from build123d import *

# Parameters (mm, degrees)
SKETCH_1_R               = 37.5
SKETCH_1_R_2             = 35.5
EXTRUDE_1_DEPTH          = 214
SKETCH_2_R               = 1.5
CUT_EXTRUDE_1_DEPTH      = 88
PATTERN_CIRCULAR_1_COUNT = 3
SKETCH_3_W               = 5
SKETCH_3_H               = 20.375275098
CUT_EXTRUDE_2_DEPTH      = 2
PATTERN_CIRCULAR_2_COUNT = 3
SKETCH_4_W               = 5
SKETCH_4_H               = 20.375275098
CUT_EXTRUDE_3_DEPTH      = 2
PATTERN_CIRCULAR_3_COUNT = 3
CUT_EXTRUDE_4_DEPTH      = 156
CUT_EXTRUDE_4_DEPTH_BACK = 165
SKETCH_5_W               = 164.762813688
SKETCH_5_H               = 214


with BuildPart() as part:
    # Эскиз1 → Бобышка-Вытянуть1 (new body)
    with BuildSketch(Plane.XY):
        Circle(SKETCH_1_R)
        Circle(SKETCH_1_R_2, mode=Mode.SUBTRACT)
    extrude(amount=EXTRUDE_1_DEPTH)

    # Эскиз2 → Вырез-Вытянуть1 (cut)
    with BuildSketch(Plane(origin=(0, 0, 0), x_dir=(1, 0, 0), z_dir=(0, 1, 0))):
        with Locations(Location((0, -5, 0), (0, 0, 270))):
            Circle(SKETCH_2_R)
        with Locations(Location((0, -209, 0), (0, 0, 270))):
            Circle(SKETCH_2_R)
    cut_extrude_1 = extrude(amount=-CUT_EXTRUDE_1_DEPTH, mode=Mode.SUBTRACT)

    # Круговой массив1: Вырез-Вытянуть1 ×3 about axis
    pattern_circular_1_axis = Axis((0, 0, 214), (0, 0, -1))
    for i in range(1, PATTERN_CIRCULAR_1_COUNT):
        add(cut_extrude_1.rotate(pattern_circular_1_axis, i * 360 / PATTERN_CIRCULAR_1_COUNT), mode=Mode.SUBTRACT)

    # Эскиз3 → Вырез-Вытянуть2 (cut)
    with BuildSketch(Plane(origin=(0, 0, 0), x_dir=(-1, 0, 0), z_dir=(0, 0, -1))):
        with Locations((0, 27.321603857)):
            Rectangle(SKETCH_3_W, SKETCH_3_H)
    cut_extrude_2 = extrude(amount=-CUT_EXTRUDE_2_DEPTH, mode=Mode.SUBTRACT)

    # Круговой массив2: Вырез-Вытянуть2 ×3 about axis
    pattern_circular_2_axis = Axis((0, 0, 0), (0, 0, 1))
    for i in range(1, PATTERN_CIRCULAR_2_COUNT):
        add(cut_extrude_2.rotate(pattern_circular_2_axis, i * 360 / PATTERN_CIRCULAR_2_COUNT), mode=Mode.SUBTRACT)

    # Эскиз4 → Вырез-Вытянуть3 (cut)
    with BuildSketch(Plane.XY.offset(214)):
        with Locations((0, 27.321603857)):
            Rectangle(SKETCH_4_W, SKETCH_4_H)
    cut_extrude_3 = extrude(amount=-CUT_EXTRUDE_3_DEPTH, mode=Mode.SUBTRACT)

    # Круговой массив3: Вырез-Вытянуть3 ×3 about axis
    pattern_circular_3_axis = Axis((0, 0, 0), (0, 0, 1))
    for i in range(1, PATTERN_CIRCULAR_3_COUNT):
        add(cut_extrude_3.rotate(pattern_circular_3_axis, i * 360 / PATTERN_CIRCULAR_3_COUNT), mode=Mode.SUBTRACT)

    # Эскиз5 → Вырез-Вытянуть4 (cut, two sides: drawn at the far end of the back side and taken through both)
    with BuildSketch(Plane(origin=(0, 0, 0), x_dir=(1, 0, 0), z_dir=(0, 1, 0)).offset(-CUT_EXTRUDE_4_DEPTH_BACK)):
        Rectangle(SKETCH_5_W, SKETCH_5_H)
    extrude(amount=CUT_EXTRUDE_4_DEPTH + CUT_EXTRUDE_4_DEPTH_BACK, mode=Mode.SUBTRACT)


solid = part.part
Could you check a few things on this model? Use its own coordinates, in mm. A direction names the side the tool comes from. Give positions to 0.01 mm unless a question says otherwise; leave off trailing zeros. Loops run counter-clockwise (first coordinate to the right, second up) from the corner with the lowest first, then second, coordinate; pieces in that order, holes last. Notation, with made-up numbers: (77, 30.25) -> (127, 30.25) arc R22 cw to (127, 67.25) -> close; hole circle Ø4 at (-30.75, -22). An arc over 180 degrees is marked (long way). Return JSON: item names as keys, results as strings.
Item 1: Which directions (+Z, -Z, +X, -X, +Y, -Y) give clear straight access to the entire face, cutting with the end or side of a thin tool? Please do faces 1 (the flat face through (-30.5, 18.6, 214)), 2 (the flat face through (32, -18, 212)), 3 (the cylindrical face through (-0.575, -36.47, 210.386)).
Geometry results:
{"face 1": "+Z, +X, -X, +Y, -Y", "face 2": "+Z", "face 3": "-Y"}
Item 2: I'm going to push flat-ended pins straight in: pin 1 (3.5 mm diameter, centred on x = 31.5, y = -17.5, fed in from +Z); pin 2 (1 mm diameter, centred on y = 8, z = 153.5, fed in from +X); pin 3 (8 mm diameter, centred on y = -27, z = 175.5, fed in from -X). Where does each tip first touch, or does it pass through?
Geometry results:
{"pin 1": "stops at z = 212", "pin 2": "stops at x = 36.74", "pin 3": "stops at x = -29.62"}
Item 3: I need wall thicknesses on L1, parallel to X at y = 0, z = 159; L2, parallel to Y at x = -9, z = 154. Which ranges of each line are inside material? Lowest first, please. Write a range as from..to.
Geometry results:
{"L1": "x = -37.5..-35.5, 35.5..37.5", "L2": "y = -36.4..-34.34, 34.34..36.4"}
Item 4: If we section it at D-D on z = 209: List the corners of the cut face in (x, y) for me.
Geometry results:
{"outline": "(-33.2, 17.44) arc R37.5 ccw to (-1.5, -37.47) -> (-1.5, -35.47) arc R35.5 cw to (-31.47, 16.44) -> close; (-31.7, 20.03) -> (-29.97, 19.03) arc R35.5 cw to (29.97, 19.03) -> (31.7, 20.03) arc R37.5 ccw to start; (1.5, -37.47) arc R37.5 ccw to (33.2, 17.44) -> (31.47, 16.44) arc R35.5 cw to (1.5, -35.47) -> close"}
Item 5: We'd pull the mould along X, two halves only. Please class faces 4 (the cylindrical face through (-4.88, 37.18, 159.75)), 5 (the flat face through (33, 14, 107)), 6 (the cylindrical face through (-31.297, 18.733, 210.386)): +X half, -X half, draft (parallel to the pull), parting line (faces both ways), or undercut.
Geometry results:
{"face 4": "parting line", "face 5": "draft", "face 6": "undercut"}
Item 6: If we section it at B-B on x = 0: List the corners of the cut face in (y, z) for me.
Geometry results:
{"outline": "(-37.5, 107) -> (-35.5, 107) -> (-35.5, 207.5) -> (-37.5, 207.5) -> close; (-37.5, 210.5) -> (-35.5, 210.5) -> (-35.5, 214) -> (-37.5, 214) -> close; (35.5, 107) -> (37.5, 107) -> (37.5, 212) -> (35.5, 212) -> close"}
Item 7: If we section it at C-C on x = -23.5: List the corners of the cut face in (y, z) for me.
Geometry results:
{"outline": "(-29.22, 107) -> (-26.61, 107) -> (-26.61, 214) -> (-29.22, 214) -> close; (26.61, 107) -> (29.22, 107) -> (29.22, 214) -> (26.61, 214) -> close"}
Item 8: If we section it at A-A on y = 0: List the corners of the cut face in (x, z) for me.
Geometry results:
{"outline": "(-37.5, 107) -> (-35.5, 107) -> (-35.5, 214) -> (-37.5, 214) -> close; (35.5, 107) -> (37.5, 107) -> (37.5, 214) -> (35.5, 214) -> close"}
